Print and shaded views of the part. All mm, measured from the part's lowest x, y and z. A direction names the side the tool comes from. Round coordinates to 2 decimals unless told otherwise and drop trailing zeros. Loops run counter-clockwise (first coordinate to the right, second up) from the corner with the lowest first, then second, coordinate; pieces in that order, holes last. Notation, with made-up numbers: (-25, 87) - (-21, 87) arc R25 cw to (-21, 123) - close; hole circle Ø6 at (68, 24.5). An arc over 180 degrees is marked (long way). Use one line per item in the form item = value. Start each with the question number.
Q1. Drill centre lines: line 1 (Y direction, x = 8, z = 6.75); line 2 (Z direction, x = 1.25, y = 3.75); line 3 (Z direction, x = 3.75, y = 3). Where is each one in solid material? Low to high.
Q2. 3-axis set-ups, long thin cutter, end or side, ignore diameter. For the marked faces 1 and 2: which of +Z, -Z, +X, -X, +Y, -Y reach the whole face in a straight line?
Q3. Saw through at B-B (x = 4.5). Give the cut face in (y, z), then the cut area to 3 significant figures.
Q4. Saw through at C-C (y = 4). Give the cut face in (x, z), then the cut area to 3 significant figures.
Q5. Pin check, flat tips, straight feed: pin 1 (5 mm diameter, centred on x = 7, y = 5, fed in from -Z); pin 2 (2 mm diameter, centred on y = 2.5, z = 1.5, fed in from +X). Stop position of each tip, or through.
Q6. Saw through at A-A (z = 4.5). Give the cut face in (x, y).
Q7. Mould opens along X. For the marked faces 3 and 4 say: released by +X, released by -X, zero draft, split by the parting line, or undercut.
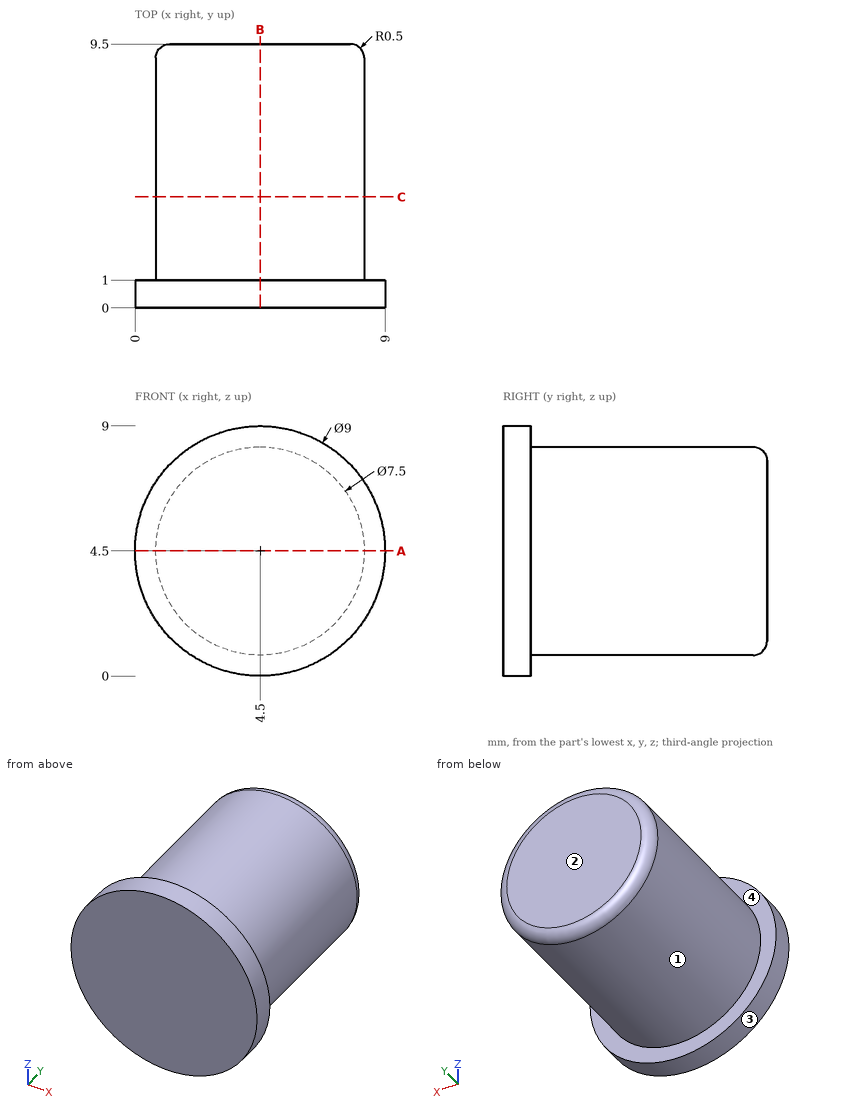
Report:
q1.line_1 = 0 to 1
q1.line_2 = 2.63 to 6.37
q1.line_3 = 0.83 to 8.17
q2.face_1 = +Y
q2.face_2 = +Z, -Z, +X, -X, +Y
q3.outline = (0, 0) - (1, 0) - (1, 0.75) - (9, 0.75) arc R0.5 ccw to (9.5, 1.25) - (9.5, 7.75) arc R0.5 ccw to (9, 8.25) - (1, 8.25) - (1, 9) - (0, 9) - close
q3.area = 72.6 mm²
q4.outline = circle Ø7.5 at (4.5, 4.5)
q4.area = 44.2 mm²
q5.pin_1 = 0.75
q5.pin_2 = 7.67
q6.outline = (0, 0) - (9, 0) - (9, 1) - (8.25, 1) - (8.25, 9) arc R0.5 ccw to (7.75, 9.5) - (1.25, 9.5) arc R0.5 ccw to (0.75, 9) - (0.75, 1) - (0, 1) - close
q7.face_3 = split by the parting line
q7.face_4 = zero draft
